Verification items for the finished model (mm, model axes). Give positions to 0.01 mm unless a question says otherwise; leave off trailing zeros. Order: outer loops, then holes, each group sorted by start corner. A loop starts at its lowest first (then second) coordinate and runs counter-clockwise, first axis right, second up. Notation, with made-up numbers: (33, 32) -> (89, 32) arc R15 cw to (89, 59) -> close; hole circle Ø1 at (31.25, 8). An arc over 180 degrees is marked (long way). Write each question's results on one line, items separated by ' | '. Start each with the question number.
1. Cross-section at A-A, the plane z = 0. Enter the section's corners in (x, y), then the cut area to 3 significant figures.
2. Depth check by flat-ended pin: pin 1 Ø10 at (x, z) = (0, 0) entering from -Y. Enter the tip coordinate at first touch or a pass-through.
3. Cross-section at C-C, the plane y = 40.4. Enter the section's corners in (x, z).
4. Material ranges on L1, parallel to X at y = 40.25, z = 0; L2, parallel to X at y = 40.35, z = -2, recorded low to high. Write a range as from..to.
5. Cross-section at B-B, the plane x = 0. Enter the section's corners in (y, z), then the cut area to 3 significant figures.
6. Mould release check, pull along X, two halves, no side actions. Record for faces 1 (the face through (-0.2, 40.5, 17.5)), 2 (the face through (0.931, 40.507, 2.957)), 3 (the face through (17.5, 40.5, 0.2)): +X half, -X half, draft (parallel to the pull), parting line (faces both ways), or undercut.
from build123d import *

# Parameters (mm, degrees)
SKETCH2_W                = 35
SKETCH2_H                = 35
BOSS_EXTRUDE1_DEPTH      = 10
SKETCH3_W                = 35
SKETCH3_H                = 35
SKETCH3_W_2              = 25
SKETCH3_H_2              = 25
BOSS_EXTRUDE2_DEPTH      = 15
SKETCH4_W                = 35
SKETCH4_H                = 35
BOSS_EXTRUDE3_DEPTH      = 15
CUT_EXTRUDE1_START       = -40
SKETCH5_R                = 3.05
CUT_EXTRUDE1_DEPTH       = 40
BOSS_EXTRUDE4_DEPTH      = 10
BOSS_EXTRUDE4_DEPTH_BACK = 40
SKETCH6_W                = 7.5
SKETCH6_H                = 1.017843133
SKETCH6_H_2              = 1.2761833
SKETCH7_R                = 2.76
CUT_EXTRUDE2_DEPTH       = 10
SKETCH8_W                = 35
SKETCH8_H                = 35
BOSS_EXTRUDE5_DEPTH      = 1
SKETCH9_R                = 3.1
CUT_EXTRUDE3_DEPTH       = 1


with BuildPart() as part:
    # Sketch2 → Boss-Extrude1 (new body)
    with BuildSketch(Plane(origin=(0, 0, 0), x_dir=(1, 0, 0), z_dir=(0, 1, 0))):
        Rectangle(SKETCH2_W, SKETCH2_H)
    extrude(amount=BOSS_EXTRUDE1_DEPTH)


with BuildPart() as body_2:
    # Sketch3 → Boss-Extrude2 (new body)
    with BuildSketch(Plane(origin=(0, 10, 0), x_dir=(1, 0, 0), z_dir=(0, 1, 0))):
        Rectangle(SKETCH3_W, SKETCH3_H)
        Rectangle(SKETCH3_W_2, SKETCH3_H_2, mode=Mode.SUBTRACT)
    extrude(amount=BOSS_EXTRUDE2_DEPTH)


with BuildPart() as body_3:
    # Sketch4 → Boss-Extrude3 (new body)
    with BuildSketch(Plane(origin=(0, 25, 0), x_dir=(1, 0, 0), z_dir=(0, 1, 0))):
        Rectangle(SKETCH4_W, SKETCH4_H)
    extrude(amount=BOSS_EXTRUDE3_DEPTH)


with BuildPart() as cut_extrude1_tool:
    # Sketch5 → Cut-Extrude1 (new body)
    with BuildSketch(Plane(origin=(0, 40, 0), x_dir=(1, 0, 0), z_dir=(0, 1, 0)).offset(CUT_EXTRUDE1_START)):
        with Locations(Location((0, 0, 0), (0, 0, 270))):
            Circle(SKETCH5_R)
    extrude(amount=CUT_EXTRUDE1_DEPTH)


with BuildPart() as part_1:
    add(part.part)

    # Cut-Extrude1: cut by cut_extrude1_tool
    add(cut_extrude1_tool.part, mode=Mode.SUBTRACT)


with BuildPart() as body_3_1:
    add(body_3.part)

    # Cut-Extrude1: cut by cut_extrude1_tool
    add(cut_extrude1_tool.part, mode=Mode.SUBTRACT)

    # Sketch6 → Boss-Extrude4 (add, two sides: drawn at the far end of the back side and taken through both)
    with BuildSketch(Plane(origin=(0, 0, -17.5), x_dir=(-1, 0, 0), z_dir=(0, 0, -1)).offset(-BOSS_EXTRUDE4_DEPTH_BACK)):
        with Locations((-13.75, 25.508921566)):
            Rectangle(SKETCH6_W, SKETCH6_H)
        with Locations((13.75, 25.63809165)):
            Rectangle(SKETCH6_W, SKETCH6_H_2)
    extrude(amount=BOSS_EXTRUDE4_DEPTH + BOSS_EXTRUDE4_DEPTH_BACK)

    # Sketch7 → Cut-Extrude2 (cut)
    with BuildSketch(Plane(origin=(0, 26.2761833, 0), x_dir=(1, 0, 0), z_dir=(0, 1, 0))):
        with Locations(Location((-13.75, 22.5, 0), (0, 0, 270))):
            Circle(SKETCH7_R)
        with Locations((8.75, 22.5)):
            Circle(SKETCH7_R)
        with Locations((8.75, -18)):
            Circle(SKETCH7_R)
        with Locations(Location((-13.75, -18, 0), (0, 0, 270))):
            Circle(SKETCH7_R)
    extrude(amount=-CUT_EXTRUDE2_DEPTH, mode=Mode.SUBTRACT)


with BuildPart() as body_2_2:
    # Sketch8 → Boss-Extrude5 (new body)
    with BuildSketch(Plane(origin=(0, 40, 0), x_dir=(1, 0, 0), z_dir=(0, 1, 0))):
        Rectangle(SKETCH8_W, SKETCH8_H)
    extrude(amount=BOSS_EXTRUDE5_DEPTH)

    # Sketch9 → Cut-Extrude3 (cut)
    with BuildSketch(Plane(origin=(0, 41, 0), x_dir=(1, 0, 0), z_dir=(0, 1, 0))):
        with Locations(Location((0, 0, 0), (0, 0, 270))):
            Circle(SKETCH9_R)
    extrude(amount=-CUT_EXTRUDE3_DEPTH, mode=Mode.SUBTRACT)


solid = body_2_2.part
Results below:
1) outline: (-17.5, 40) -> (-3.1, 40) -> (-3.1, 41) -> (-17.5, 41) -> close; (3.1, 40) -> (17.5, 40) -> (17.5, 41) -> (3.1, 41) -> close | area: 28.8 mm²
2) pin 1: stops at y = 40
3) outline: (-17.5, -17.5) -> (17.5, -17.5) -> (17.5, 17.5) -> (-17.5, 17.5) -> close; hole circle Ø6.2 at (0, 0)
4) L1: x = -17.5..-3.1, 3.1..17.5 | L2: x = -17.5..-2.37, 2.37..17.5
5) outline: (40, -17.5) -> (41, -17.5) -> (41, -3.1) -> (40, -3.1) -> close; (40, 3.1) -> (41, 3.1) -> (41, 17.5) -> (40, 17.5) -> close | area: 28.8 mm²
6) face 1: draft | face 2: undercut | face 3: +X half
